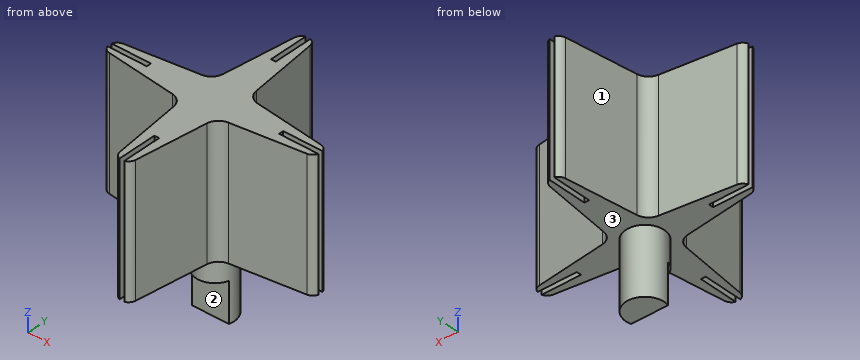
```python
from build123d import *

# Parameters (mm, degrees)
BOSS_EXTRUDE1_DEPTH = 49
FILLET1_R           = 5
SKETCH2_R           = 7.25
BOSS_EXTRUDE2_DEPTH = 25
CUT_EXTRUDE1_START  = -15
CUT_EXTRUDE1_DEPTH  = 15
SKETCH4_W           = 25
SKETCH4_H           = 1.7875
SKETCH4_W_2         = 1.7875
SKETCH4_H_2         = 25
CUT_EXTRUDE2_DEPTH  = 49


with BuildPart() as part:
    # Sketch1 → Boss-Extrude1 (new body)
    with BuildSketch(Plane.XY):
        with BuildLine():
            Line((-6.731298149, 6.731298149), (-2.97772961, 37.364864865))
            ThreePointArc((-2.97772961, 37.364864865), (0, 40), (2.97772961, 37.364864865))
            Line((2.97772961, 37.364864865), (6.731298149, 6.731298149))
            Line((6.731298149, 6.731298149), (37.364864865, 2.97772961))
            ThreePointArc((37.364864865, 2.97772961), (40, 0), (37.364864865, -2.97772961))
            Line((37.364864865, -2.97772961), (6.731298149, -6.731298149))
            Line((6.731298149, -6.731298149), (2.97772961, -37.364864865))
            ThreePointArc((2.97772961, -37.364864865), (0, -40), (-2.97772961, -37.364864865))
            Line((-2.97772961, -37.364864865), (-6.731298149, -6.731298149))
            Line((-6.731298149, -6.731298149), (-37.364864865, -2.97772961))
            ThreePointArc((-37.364864865, -2.97772961), (-40, 0), (-37.364864865, 2.97772961))
            Line((-37.364864865, 2.97772961), (-6.731298149, 6.731298149))
        make_face()
    extrude(amount=BOSS_EXTRUDE1_DEPTH)

    # Fillet1
    fillet1_edges = [part.edges().sort_by_distance(p)[0] for p in [
        (-6.731298149, 6.731298149, 24.5),
        (6.731298149, 6.731298149, 24.5),
        (6.731298149, -6.731298149, 24.5),
        (-6.731298149, -6.731298149, 24.5),
    ]]
    fillet(fillet1_edges, radius=FILLET1_R)

    # Sketch2 → Boss-Extrude2 (add)
    with BuildSketch(Plane(origin=(0, 0, 0), x_dir=(-1, 0, 0), z_dir=(0, 0, -1))):
        with Locations(Location((0, 0, 0), (0, 0, 180))):
            Circle(SKETCH2_R)
    extrude(amount=BOSS_EXTRUDE2_DEPTH)

    # Sketch3 → Cut-Extrude1 (cut)
    with BuildSketch(Plane(origin=(0, 0, -25), x_dir=(-1, 0, 0), z_dir=(0, 0, -1)).offset(CUT_EXTRUDE1_START)):
        with BuildLine():
            Line((6.968679932, -2), (-6.968679932, -2))
            ThreePointArc((-6.968679932, -2), (0, -7.25), (6.968679932, -2))
        make_face()
    extrude(amount=CUT_EXTRUDE1_DEPTH, mode=Mode.SUBTRACT)

    # Sketch4 → Cut-Extrude2 (cut)
    with BuildSketch(Plane.XY.offset(49)):
        with Locations((37.5, 0)):
            Rectangle(SKETCH4_W, SKETCH4_H)
        with Locations((0, 37.5)):
            Rectangle(SKETCH4_W_2, SKETCH4_H_2)
        with Locations((0, -37.5)):
            Rectangle(SKETCH4_W_2, SKETCH4_H_2)
        with Locations((-37.5, 0)):
            Rectangle(SKETCH4_W, SKETCH4_H)
    extrude(amount=-CUT_EXTRUDE2_DEPTH, mode=Mode.SUBTRACT)


solid = part.part
```
Model file for the job. Use its own axes, mm. Face numbers are marked on the shaded views. A direction names the side the tool comes from. Coordinates: 2 decimals unless noted, no trailing zeros. Order: outer loops, then holes, each group sorted by start corner. A loop starts at its lowest first (then second) coordinate and runs counter-clockwise, first axis right, second up. Notation, with made-up numbers: (6, -33.5) - (30, -33.5) arc R34 cw to (30, 0.5) - close; hole circle Ø8 at (-9.5, 87). An arc over 180 degrees is marked (long way). Return JSON: item names as keys, results as strings. Group by question number.
1) Probe line 1 (X direction, y = -29.5, z = 41); line 2 (Y direction, x = -28, z = 3); line 3 (Z direction, x = -1, y = -29). List the from-to ranges inside material, lowest first. Write a range as from..to.
2) Saw through at C-C, the plane x = 13. Write the cut outline in (y, z), plus the area to 3 significant figures.
3) Flat gauge pins, fed straight in: P1, Ø1.5, axis at x = -13.5, z = 18, coming from the +Y side; P2, Ø4, axis at x = 21.5, z = 26.5, coming from the -Y side; P3, Ø12, axis at x = 29, z = 27.5, coming from the -Y side. Where does each tip first touch, or does it go through?
4) Tool access for the marked faces 1, 2 and 3: list every direction of +Z, -Z, +X, -X, +Y, -Y with a clear straight run to the whole face (end or side of a thin tool).
5) Saw through at D-D, the plane x = -14. Write the cut outline in (y, z).
6) Saw through at B-B, the plane y = 33. Write the cut outline in (x, z), plus the area to 3 significant figures.
Values found:
{
 "1": {"line 1": "x = -3.94..-0.89, 0.89..3.94", "line 2": "y = -4.13..-0.89, 0.89..4.13", "line 3": "z = 0..49"},
 "2": {"outline": "(-5.96, 0) - (5.96, 0) - (5.96, 49) - (-5.96, 49) - close", "area": "584 mm²"},
 "3": {"P1": "stops at y = 5.99", "P2": "stops at y = -5.17", "P3": "stops at y = -4.74"},
 "4": {"face 1": "+Z, -Z, -X, +Y", "face 2": "-Z, +X, -X, -Y", "face 3": "-Z"},
 "5": {"outline": "(-5.84, 0) - (5.84, 0) - (5.84, 49) - (-5.84, 49) - close"},
 "6": {"outline": "(-3.51, 0) - (-0.89, 0) - (-0.89, 49) - (-3.51, 49) - close; (0.89, 0) - (3.51, 0) - (3.51, 49) - (0.89, 49) - close", "area": "257 mm²"}
}
